For this review, take the finished solid that the model builds, in its own axes (mm). Give positions to 0.01 mm unless a question says otherwise; leave off trailing zeros. Order: outer loops, then holes, each group sorted by start corner. A loop starts at its lowest first (then second) coordinate and runs counter-clockwise, first axis right, second up.
Item 1: For P1, Ø1.5, axis at x = 35.5, z = -2.5, coming from the -Y side, flat-tipped, find the tip position at first contact; note if it passes through.
Item 2: Consider section A-A (x = 35.5). Give the boundary of the cut face in (y, z), plus the area to 3 significant figures.
Item 3: The part is to be moulded in two halves that separate along Z. For faces 1 (the flat face through (19, 0, -33)), 2 (the cylindrical face through (4.58, 0.51, -3.27)), say which applies: released by +Z, released by -Z, zero draft, split by the parting line, or undercut.
Item 4: For probe 1 along Z at (x, y) = (36.5, 0.45); probe 2 along Z at (x, y) = (35, 0.95), list the stretches that pass through material, from the lowest coordinate up.
```python
from build123d import *

# Parameters (mm, degrees)
SKETCH1_W           = 38
SKETCH1_H           = 66
BOSS_EXTRUDE1_DEPTH = 1
SKETCH2_R           = 1.25
CUT_EXTRUDE1_DEPTH  = 2
SKETCH3_R           = 0.456831937
SKETCH3_R_2         = 0.409961783
SKETCH3_R_3         = 0.739914173
SKETCH3_R_4         = 0.716276255
CUT_EXTRUDE2_DEPTH  = 2


with BuildPart() as part:
    # Sketch1 → Boss-Extrude1 (new body)
    with BuildSketch(Plane(origin=(0, 0, 0), x_dir=(1, 0, 0), z_dir=(0, 1, 0))):
        with Locations((19, 33)):
            Rectangle(SKETCH1_W, SKETCH1_H)
    extrude(amount=BOSS_EXTRUDE1_DEPTH)

    # Sketch2 → Cut-Extrude1 (cut, through all)
    with BuildSketch(Plane(origin=(0, 1, 0), x_dir=(1, 0, 0), z_dir=(0, 1, 0))):
        with Locations((35.5, 2.5)):
            Circle(SKETCH2_R)
    extrude(amount=-CUT_EXTRUDE1_DEPTH, mode=Mode.SUBTRACT)

    # Sketch3 → Cut-Extrude2 (cut, through all)
    with BuildSketch(Plane(origin=(0, 1, 0), x_dir=(1, 0, 0), z_dir=(0, 1, 0))):
        with Locations((2.638016887, 4.098772659)):
            Circle(SKETCH3_R)
        with Locations((2.638016887, 8.613282996)):
            Circle(SKETCH3_R_2)
        with Locations((5.107560434, 9.90998851)):
            Circle(SKETCH3_R_3)
        with Locations((5.107560434, 2.785166116)):
            Circle(SKETCH3_R_4)
    extrude(amount=-CUT_EXTRUDE2_DEPTH, mode=Mode.SUBTRACT)


solid = part.part
```
Resolved:
1. P1: passes through
2. outline: (0, -66) - (1, -66) - (1, -3.75) - (0, -3.75) - close; (0, -1.25) - (1, -1.25) - (1, 0) - (0, 0) - close
2. area: 63.5 mm2
3. face 1: zero draft
3. face 2: undercut
4. probe 1: z = -66 to -3.25, -1.75 to 0
4. probe 2: z = -66 to -3.65, -1.35 to 0
